For this review, take the finished solid that the model builds, in its own axes (mm). Face numbers are marked on the shaded views. Round coordinates to 2 decimals unless told otherwise and drop trailing zeros. Loops run counter-clockwise (first coordinate to the right, second up) from the corner with the lowest first, then second, coordinate; pieces in that order, holes last. Notation, with made-up numbers: (-9.5, -18.75) -> (23.5, -18.75) arc R25 ccw to (23.5, 20.25) -> close; hole circle Ø10 at (-28, 16.5). An arc over 180 degrees is marked (long way). One line per question, with ' | ' between items. Start each with the question number.
1. Consider section B-B (z = 6.3). Write out the cut boundary in (x, y), and give its area (3 significant figures).
2. Consider section A-A (x = 6.3). Write out the cut boundary in (y, z) (3 decimals), and give its area (3 significant figures).
3. Draft analysis for pull direction Y (two halves, no side actions). For the marked faces 1, 2, 3 and 4, state which applies: pulls with the +Y half, pulls with the -Y half, needs draft (parallel to the pull), parting line crosses it, or undercut.
4. Consider section D-D (x = 1). Write out the cut boundary in (y, z) (3 decimals).
5. Wall thickness on line 1 along X through (y, z) = (5, 6); line 2 along Y through (x, z) = (7.75, 0.75); line 3 along Y through (x, z) = (3, 3.25): over which ranges is each line inside the solid? List them lowest first.
6. For pin 1 Ø1 at (x, y) = (9.5, 11.5) entering from -Z; pin 2 Ø2.5 at (x, y) = (6.3, 75) entering from -Z, all flat-tipped, find the tip position at first contact; note any pin that passes through.
7. Consider section C-C (y = 33). Write out the cut boundary in (x, z), and give its area (3 significant figures).
Autodesk Inventor part; units mm, degrees
ref_plane "YZ Plane" through (0, 0, 0) normal (1, 0, 0) x (0, 1, 0)
ref_plane "XZ Plane" through (0, 0, 0) normal (0, 1, 0) x (-1, 0, 0)
ref_plane "XY Plane" through (0, 0, 0) normal (0, 0, 1) x (1, 0, 0)
sketch "Szkic1" plane through (0, 0, 0) normal (0, 0, 1) x (1, 0, 0)
  point P0 (0, 0)
sketch "Szkic2" plane through (0, 0, 0) normal (0, 1, 0) x (-1, 0, 0)
  line L0 (0, 0) -> (-12.6, 0)
  line L1 (-12.6, 0) -> (-12.6, 12.6)
  line L2 (-12.6, 12.6) -> (0, 12.6)
  line L3 (0, 12.6) -> (0, 0)
  dimension "d0" = 12.6
  dimension "d1" = 12.6
extrude "Wyciągnięcie proste1" add sketch "Szkic2" along normal blind 80
sketch "Szkic3" plane through (12.6, 0, 12.6) normal (1, 0, 0) x (0, 0, -1)
  line L0 (12.6, 0) -> (0, 0)
  line L1 (12.6, 0) -> (12.6, 80)
  line L2 (0, 80) -> (12.6, 80)
  line L3 (0, 0) -> (0, 80)
  arc A0 (5.1341, 38.375) -> (7.4659, 38.375) centre (6.3, 33) ccw
  arc A1 (7.4659, 41.625) -> (5.1341, 41.625) centre (6.3, 47) ccw
  arc A2 (5.1341, 41.625) -> (5.1341, 38.375) centre (6.3, 40) ccw
  arc A3 (7.4659, 38.375) -> (7.4659, 41.625) centre (6.3, 40) ccw
  dimension "d5" = 11
  dimension "d6" = 33
  dimension "d7" = 11
  dimension "d8" = 33
extrude "Wyciągnięcie proste2" cut sketch "Szkic3" against normal blind 80 contours A2 A1 A3 A0
sketch "Szkic4" plane through (0, 0, 12.6) normal (0, 0, 1) x (1, 0, 0)
  line L0 (12.6, 27.5) -> (0, 27.5)
  line L1 (12.6, 0) -> (0, 0)
  line L2 (12.6, 0) -> (12.6, 80)
  line L3 (0, 80) -> (12.6, 80)
  line L4 (0, 0) -> (0, 80)
  point P0 (6.3, 5)
  point P1 (6.3, 20)
  point P2 (6.3, 60)
  point P3 (6.3, 75)
  dimension "d11" = 5
  dimension "d12" = 15
  dimension "d13" = 5
  dimension "d15" = 15
hole "Otwór1" at (6.3, 5, 12.6) at (6.3, 20, 12.6) direction (0, 0, -1) diameter 3.5 end through all
hole "Otwór2" at (6.3, 60, 12.6) at (6.3, 75, 12.6) direction (0, 0, -1) diameter 4.3 end through all
properties part number "belka_tensometryczna"
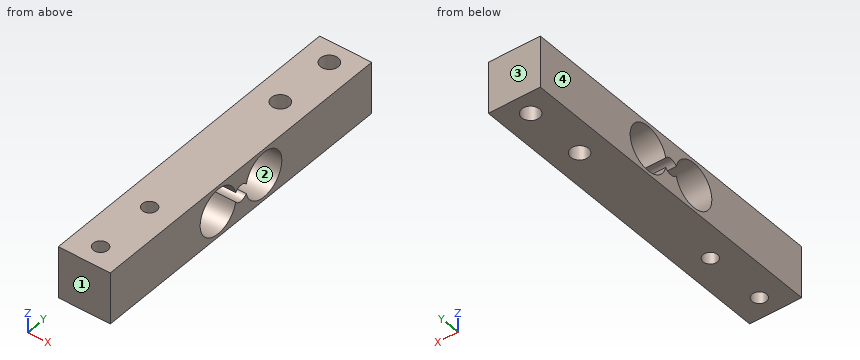
Answer block:
1) outline: (0, 0) -> (12.6, 0) -> (12.6, 27.5) -> (0, 27.5) -> close; (0, 52.5) -> (12.6, 52.5) -> (12.6, 80) -> (0, 80) -> close; hole circle Ø4.3 at (6.3, 60); hole circle Ø4.3 at (6.3, 75); hole circle Ø3.5 at (6.3, 5); hole circle Ø3.5 at (6.3, 20) | area: 645 mm2
2) outline: (0, 0) -> (3.25, 0) -> (3.25, 12.6) -> (0, 12.6) -> close; (6.75, 0) -> (18.25, 0) -> (18.25, 12.6) -> (6.75, 12.6) -> close; (21.75, 0) -> (57.85, 0) -> (57.85, 12.6) -> (21.75, 12.6) -> close; (62.15, 0) -> (72.85, 0) -> (72.85, 12.6) -> (62.15, 12.6) -> close; (77.15, 0) -> (80, 0) -> (80, 12.6) -> (77.15, 12.6) -> close; hole (38.375, 5.134) arc R2 ccw to (41.625, 5.134) arc R5.5 ccw (long way) to (41.625, 7.466) arc R2 ccw to (38.375, 7.466) arc R5.5 ccw (long way) to start | area: 610 mm2
3) face 1: pulls with the -Y half | face 2: undercut | face 3: pulls with the +Y half | face 4: needs draft
4) outline: (0, 0) -> (80, 0) -> (80, 12.6) -> (0, 12.6) -> close; hole (38.375, 5.134) arc R2 ccw to (41.625, 5.134) arc R5.5 ccw (long way) to (41.625, 7.466) arc R2 ccw to (38.375, 7.466) arc R5.5 ccw (long way) to start
5) line 1: x = 0 to 4.55, 8.05 to 12.6 | line 2: y = 0 to 4.02, 5.98 to 19.02, 20.98 to 58.41, 61.59 to 73.41, 76.59 to 80 | line 3: y = 0 to 28.42, 37.58 to 42.42, 51.58 to 80
6) pin 1: stops at z = 0 | pin 2: passes through
7) outline: (0, 0) -> (12.6, 0) -> (12.6, 0.8) -> (0, 0.8) -> close; (0, 11.8) -> (12.6, 11.8) -> (12.6, 12.6) -> (0, 12.6) -> close | area: 20.2 mm2
